```python
from build123d import *

# Parameters (mm, degrees)
ESBO_O1_R                = 14.2875
ESBO_O1_R_2              = 2.6
RESSALTO_EXTRUS_O2_DEPTH = 4
FILETE1_R                = 15
ESBO_O3_R                = 1.5
ESBO_O3_R_2              = 2.6
ESBO_O3_R_3              = 3.05
CORTE_EXTRUS_O1_DEPTH    = 5
ESBO_O5_R                = 2.25
ESBO_O5_R_2              = 3
ESBO_O5_R_3              = 1.6
ESBO_O5_R_4              = 2.6
CORTE_EXTRUS_O2_DEPTH    = 5


with BuildPart() as part:
    # Esboço1 → Ressalto-extrusão2 (new body)
    with BuildSketch(Plane.XY):
        Polygon((0, 0), (0, 215), (50, 215), (100, 0), align=None)
        with Locations((25, 195)):
            Circle(ESBO_O1_R, mode=Mode.SUBTRACT)
        with Locations((9.5, 14.5)):
            Circle(ESBO_O1_R_2, mode=Mode.SUBTRACT)
        with BuildLine():
            Line((20, 95), (20, 66))
            ThreePointArc((20, 66), (20.878679656, 63.878679656), (23, 63))
            Line((23, 63), (61.03739436, 63))
            ThreePointArc((61.03739436, 63), (63.386715693, 64.134339454), (63.959418441, 66.679540484))
            Line((63.959418441, 66.679540484), (57.215232395, 95.679540484))
            ThreePointArc((57.215232395, 95.679540484), (56.15886886, 97.349321333), (54.293208314, 98))
            Line((54.293208314, 98), (23, 98))
            ThreePointArc((23, 98), (20.878679656, 97.121320344), (20, 95))
        make_face(mode=Mode.SUBTRACT)
        with BuildLine():
            Line((20, 40), (20, 23))
            ThreePointArc((20, 23), (20.878679656, 20.878679656), (23, 20))
            Line((23, 20), (71.03739436, 20))
            ThreePointArc((71.03739436, 20), (73.386715693, 21.134339454), (73.959418441, 23.679540484))
            Line((73.959418441, 23.679540484), (70.005930069, 40.679540484))
            ThreePointArc((70.005930069, 40.679540484), (68.949566534, 42.349321333), (67.083905988, 43))
            Line((67.083905988, 43), (23, 43))
            ThreePointArc((23, 43), (20.878679656, 42.121320344), (20, 40))
        make_face(mode=Mode.SUBTRACT)
    extrude(amount=RESSALTO_EXTRUS_O2_DEPTH)

    # Filete1
    filete1_edges = [part.edges().sort_by_distance(p)[0] for p in [
        (0, 215, 2),
        (50, 215, 2),
    ]]
    fillet(filete1_edges, radius=FILETE1_R)

    # Esboço3 → Corte-extrusão1 (cut, through all)
    with BuildSketch(Plane(origin=(0, 0, 0), x_dir=(-1, 0, 0), z_dir=(0, 0, -1))):
        with Locations((-9.5, 112)):
            Circle(ESBO_O3_R)
        with Locations((-90.5, 14.5)):
            Circle(ESBO_O3_R_2)
        with Locations((-9.5, 137)):
            Circle(ESBO_O3_R)
        with Locations((-9.5, 152)):
            Circle(ESBO_O3_R_3)
        with Locations((-59, 112)):
            Circle(ESBO_O3_R)
    extrude(amount=-CORTE_EXTRUS_O1_DEPTH, mode=Mode.SUBTRACT)

    # Esboço5 → Corte-extrusão2 (cut, through all)
    with BuildSketch(Plane(origin=(0, 0, 0), x_dir=(-1, 0, 0), z_dir=(0, 0, -1))):
        with Locations((-25, 171.1875)):
            Circle(ESBO_O5_R)
        with Locations((-70.759810426, 80.398555206)):
            Circle(ESBO_O5_R_2)
        with Locations((-20, 162.1875)):
            Circle(ESBO_O5_R_3)
        with Locations((-48, 162.1875)):
            Circle(ESBO_O5_R_3)
        with Locations((-45, 195)):
            Circle(ESBO_O5_R_4)
        with Locations((-5, 195)):
            Circle(ESBO_O5_R_4)
    extrude(amount=-CORTE_EXTRUS_O2_DEPTH, mode=Mode.SUBTRACT)


solid = part.part
```
Design review of the part built by this model. Coordinates are the model's own, in mm. A direction names the side the tool comes from. Round coordinates to 2 decimals unless told otherwise and drop trailing zeros. Write each loop counter-clockwise with the first axis right and the second up, starting at its lowest first coordinate (ties: lowest second). Pieces come first, ordered by that corner, then holes.
Item 1: The part is to be moulded in two halves that separate along Y. For faces 3 (the cylindrical face through (23.962, 169.191, 1.972)), 4 (the cylindrical face through (47.31, 211.83, 2.03)), 5 (the flat face through (0, 99, 2)), say which applies: +Y half, -Y half, draft (parallel to the pull), parting line (faces both ways), or undercut.
Item 2: Clearance check with flat-ended pins moving along their axes: pin 1 Ø1.2 at (y, z) = (85.5, 2) entering from +X; pin 2 Ø1.2 at (x, z) = (46.5, 2) entering from -Y; pin 3 Ø1.2 at (x, z) = (45, 2.5) entering from +Y. State where each tip first meets the part, or that it passes through.
Item 3: We need section D-D on z = 1.55. State how many separate pieces and enclosed holes the cut face has, and give its area (3 significant figures).
Item 4: For probe 1 along Y at (x, z) = (23.5, 3.6); probe 2 along Y at (x, z) = (9.5, 0.95); probe 3 along Y at (x, z) = (45, 1.8), list the stretches that pass through material, from the lowest coordinate up.
Item 5: We need section B-B on y = 152. Write out the cut boundary in (x, z).
Item 6: We need section C-C on x = 31. Write out the cut boundary in (y, z).
Item 7: We need section A-A on y = 195. Write out the cut boundary in (x, z).
Item 8: For faces 1 (the flat face through (40, 109, 4)), 2 (the flat face through (72, 32.1, 2)), list the 3-axis set-ups (+Z, -Z, +X, -X, +Y, -Y) from which the entire face can be reached by the end or side of a thin tool; tool diameter is ignored.
Returned:
1. face 3: undercut
1. face 4: +Y half
1. face 5: draft
2. pin 1: stops at x = 80.26
2. pin 2: stops at y = 0
2. pin 3: stops at y = 213.61
3. separate pieces: 1
3. enclosed holes: 15
3. area: 12,600 mm2
4. probe 1: y = 0 to 20, 43 to 63, 98 to 169.51, 172.86 to 180.79, 209.21 to 215
4. probe 2: y = 0 to 11.9, 17.1 to 110.5, 113.5 to 135.5, 138.5 to 148.95, 155.05 to 213.96
4. probe 3: y = 0 to 20, 43 to 63, 98 to 192.4, 197.6 to 213.31
5. outline: (0, 0) - (6.45, 0) - (6.45, 4) - (0, 4) - close; (12.55, 0) - (64.65, 0) - (64.65, 4) - (12.55, 4) - close
6. outline: (0, 0) - (20, 0) - (20, 4) - (0, 4) - close; (43, 0) - (63, 0) - (63, 4) - (43, 4) - close; (98, 0) - (182.03, 0) - (182.03, 4) - (98, 4) - close; (207.97, 0) - (215, 0) - (215, 4) - (207.97, 4) - close
7. outline: (0, 0) - (2.4, 0) - (2.4, 4) - (0, 4) - close; (7.6, 0) - (10.71, 0) - (10.71, 4) - (7.6, 4) - close; (39.29, 0) - (42.4, 0) - (42.4, 4) - (39.29, 4) - close; (47.6, 0) - (54.65, 0) - (54.65, 4) - (47.6, 4) - close
8. face 1: +Z, +X, -X, +Y, -Y
8. face 2: +Z, -Z
